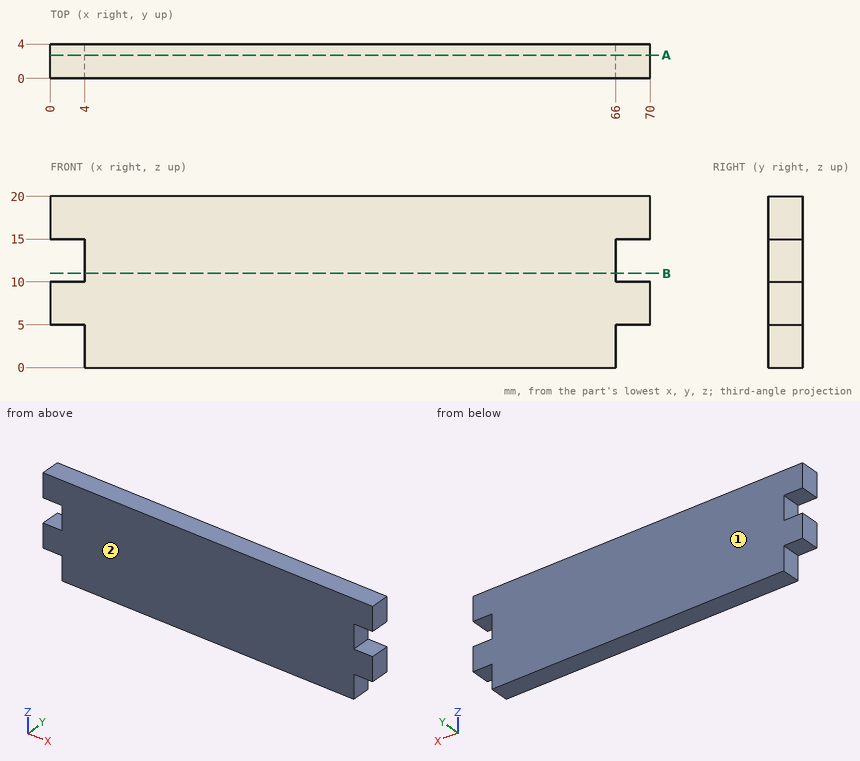
Could you check a few things on this drawing? It's one solid part, dimensions in mm from its lowest x, y, z. Round coordinates to 2 decimals unless told otherwise and drop trailing zeros. Order: outer loops, then holes, each group sorted by start corner. A loop starts at its lowest first (then second) coordinate and runs counter-clockwise, first axis right, second up. Notation, with made-up numbers: M -31,41.5 L 4,41.5 A4 ccw 4,47.5 Z; hole C 19,-8 d11. An arc over 180 degrees is marked long. One line per question, with ' | ' between items.
1) Imagine slicing it at A-A, the plane y = 2.7. Write out the boundary of the cut face in (x, z).
Checked values:
outline: M 0,5 L 4,5 L 4,0 L 66,0 L 66,5 L 70,5 L 70,10 L 66,10 L 66,15 L 70,15 L 70,20 L 0,20 L 0,15 L 4,15 L 4,10 L 0,10 Z
2) Imagine slicing it at B-B, the plane z = 11. Write out the boundary of the cut face in (x, y).
Checked values:
outline: M 4,0 L 66,0 L 66,4 L 4,4 Z
3) We'd pull the mould along Y, two halves only. Please class the marked faces 1 and 2: released by +Y, released by -Y, zero draft, split by the parting line, or undercut.
Checked values:
face 1: released by +Y | face 2: released by -Y
4) I need wall thicknesses on line 1 (X direction, y = 0.35, z = 11). Which ranges of the line are inside material? Lowest first, please.
Checked values:
line 1: x = 4 to 66
5) I'm going to push flat-ended pins straight in: pin 1 Ø1 at (y, z) = (1.5, 3) entering from -X; pin 2 Ø1.2 at (x, y) = (2.5, 2) entering from -Z; pin 3 Ø1.2 at (y, z) = (1, 13.5) entering from +X. Where does each tip first touch, or does it pass through?
Checked values:
pin 1: stops at x = 4 | pin 2: stops at z = 5 | pin 3: stops at x = 66
